Part print with two shaded views. Sizes in mm from the minimum x, y, z corner. A direction names the side the tool comes from. Round coordinates to 2 decimals unless told otherwise and drop trailing zeros. Write each loop counter-clockwise with the first axis right and the second up, starting at its lowest first coordinate (ties: lowest second). Pieces come first, ordered by that corner, then holes. Notation, with made-up numbers: M 22.5,-4 L 38.5,-4 A19 ccw 38.5,11 Z; hole C -40,52.5 d9. An arc over 180 degrees is marked long. One line per question, with ' | ' between items. Start each with the question number.
1) Saw through at A-A (x = 30). List the corners of the cut face in (y, z).
2) Mould opens along Y. For the marked faces 3, 4, 5 and 6 say: pulls with the +Y half, pulls with the -Y half, needs draft (parallel to the pull), parting line crosses it, or undercut.
3) Saw through at B-B (z = 12.5). List the corners of the cut face in (x, y), plus the area to 3 significant figures.
4) Saw through at C-C (y = 30). List the corners of the cut face in (x, z).
5) Tool access for the marked faces 1 and 2: list every direction of +Z, -Z, +X, -X, +Y, -Y with a clear straight run to the whole face (end or side of a thin tool).
6) Wall check: probe 1 along Y at (x, z) = (30.5, 12) (3 decimals); probe 2 along Y at (x, z) = (30, 24); probe 3 along Z at (x, y) = (50, 31.5). Give the ranges that are in metal, low to high. Write a range as [from, to].
7) Saw through at D-D (z = 27). List the corners of the cut face in (x, y).
8) Drop flat-ended pins along their axis: pin 1 Ø2 at (x, y) = (43, 35) entering from +Z; pin 2 Ø3 at (x, z) = (47.5, 17.5) entering from +Y; pin 3 Ø6 at (x, z) = (49.5, 25.5) entering from -Y. Give the stop position or say it passes through.
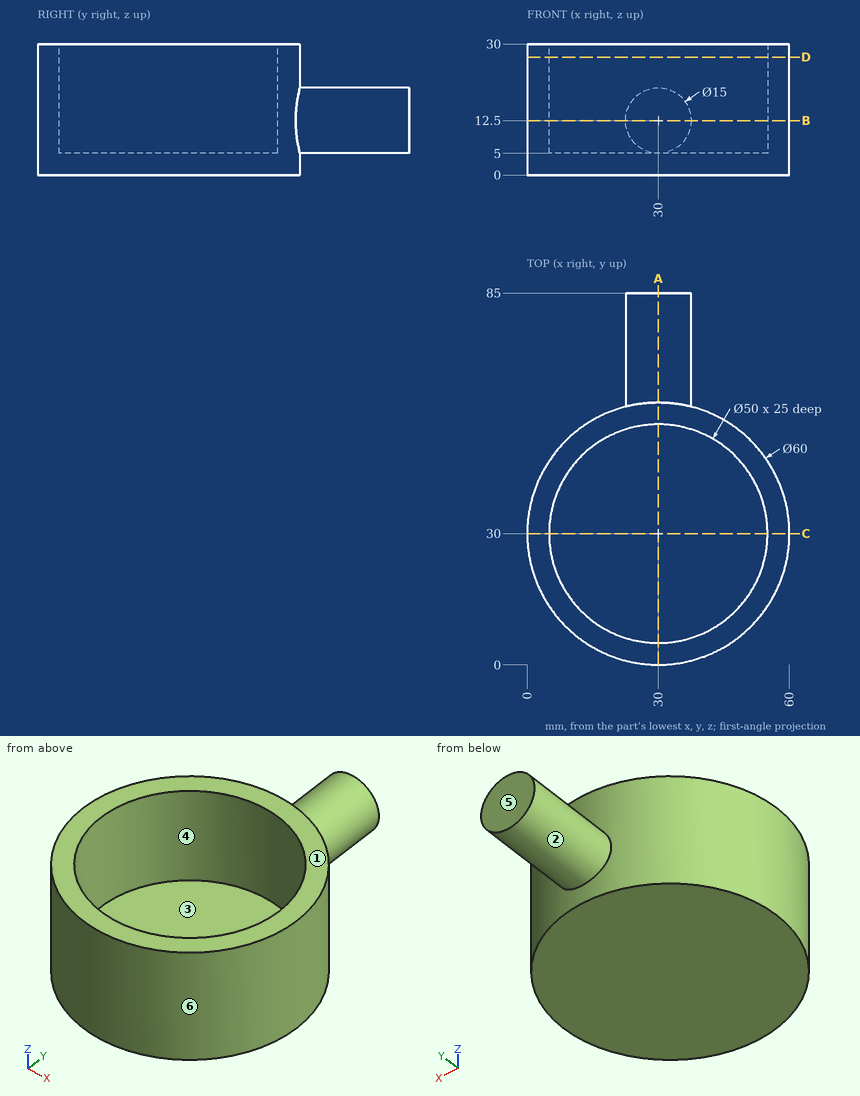
Answer key:
1) outline: M 0,0 L 60,0 L 60,5 L 85,5 L 85,20 L 60,20 L 60,30 L 55,30 L 55,5 L 5,5 L 5,30 L 0,30 Z
2) face 3: undercut | face 4: undercut | face 5: pulls with the +Y half | face 6: parting line crosses it
3) outline: M 22.5,59.05 A30 ccw long 37.5,59.05 L 37.5,85 L 22.5,85 Z; hole C 30,30 d50 | area: 1,240 mm2
4) outline: M 0,0 L 60,0 L 60,30 L 55,30 L 55,5 L 5,5 L 5,30 L 0,30 Z
5) face 1: +Z, +X, -X, +Y, -Y | face 2: +Y
6) probe 1: y = [0.004, 5.005], [54.995, 85] | probe 2: y = [0, 5], [55, 60] | probe 3: z = [0, 5]
7) outline: C 30,30 d60; hole C 30,30 d50
8) pin 1: stops at z = 5 | pin 2: stops at y = 55.38 | pin 3: stops at y = 4.95
